The listing builds one solid part. Answer for the finished solid, in the listing's coordinates (mm). Round coordinates to 2 decimals unless told otherwise and drop trailing zeros. Write each loop counter-clockwise with the first axis right and the second up, starting at its lowest first coordinate (ties: lowest second). Pieces come first, ordered by that corner, then holes. Notation, with made-up numbers: (-39, -2) - (13, -2) arc R12 ccw to (13, 3) - close; hole circle Ø7 at (55.25, 30.25). An arc over 180 degrees is marked (long way). Use a Markdown table: item, result. Add a question column.
1) A cutting plane is placed at D-D (x = -40.25). Give the vertices of the cut face in (y, z).
2) A cutting plane is placed at C-C (z = 2.1). State how many separate pieces and enclosed holes the cut face has, then the cut area to 3 significant figures.
3) A cutting plane is placed at B-B (y = -8.75). Give the vertices of the cut face in (x, z).
4) Find the intervals of material crossed by probe 1 along Y at (x, z) = (49, 2.1); probe 2 along Y at (x, z) = (40.25, 2); probe 3 along X at (y, z) = (-7, 1.25), in increasing order. Write a range as from..to.
5) A cutting plane is placed at A-A (x = 57.75). Give the vertices of the cut face in (y, z).
6) Each of these flat-tipped pins is pushed along its axis until it touches: P1, Ø2.5, axis at x = 66.5, y = 0, coming from the -Z side; P2, Ø5, axis at x = -33.84, y = 8.75, coming from the -Z side; P3, Ø1.5, axis at x = -50.5, z = 3.5, coming from the +Y side; P4, Ø1, axis at y = 5, z = 1.5, coming from the +X side. Where does it stop, or does it pass through?
7) Determine the mould class of faces 1 (the flat face through (-1, 0, 0)), 2 (the cylindrical face through (65.634, -8.284, 2.535)), 3 (the flat face through (1, 21, 2)) for opening direction Y: +Y half, -Y half, draft (parallel to the pull), parting line (faces both ways), or undercut.
```python
from build123d import *

# Parameters (mm, degrees)
EXTRUDE_1_DEPTH     = 5
SKETCH_2_R          = 13.5
SKETCH_2_R_2        = 1.55
CUT_EXTRUDE_1_DEPTH = 5


with BuildPart() as part:
    # 草图1 → 凸台-拉伸1 (new body)
    with BuildSketch(Plane.XY):
        with BuildLine():
            Line((-49, -21), (49, -21))
            ThreePointArc((49, -21), (70, 0), (49, 21))
            Line((49, 21), (-49, 21))
            ThreePointArc((-49, 21), (-70, 0), (-49, -21))
        make_face()
    extrude(amount=EXTRUDE_1_DEPTH)

    # 草图2 → 切除-拉伸1 (cut)
    with BuildSketch(Plane.XY.offset(5)):
        with Locations((49, 0)):
            Circle(SKETCH_2_R)
        with Locations((49, 17.5)):
            Circle(SKETCH_2_R_2)
        with Locations((57.75, 15.155444566)):
            Circle(SKETCH_2_R_2)
        with Locations((64.155444566, 8.75)):
            Circle(SKETCH_2_R_2)
        with Locations((66.5, 0)):
            Circle(SKETCH_2_R_2)
        with Locations((64.155444566, -8.75)):
            Circle(SKETCH_2_R_2)
        with Locations((57.75, -15.155444566)):
            Circle(SKETCH_2_R_2)
        with Locations((49, -17.5)):
            Circle(SKETCH_2_R_2)
        with Locations((40.25, -15.155444566)):
            Circle(SKETCH_2_R_2)
        with Locations((33.844555434, -8.75)):
            Circle(SKETCH_2_R_2)
        with Locations((31.5, 0)):
            Circle(SKETCH_2_R_2)
        with Locations((33.844555434, 8.75)):
            Circle(SKETCH_2_R_2)
        with Locations((40.25, 15.155444566)):
            Circle(SKETCH_2_R_2)
    cut_extrude_1 = extrude(amount=-CUT_EXTRUDE_1_DEPTH, mode=Mode.SUBTRACT)

    # 镜向1: 切除-拉伸1 across plane
    add(cut_extrude_1.mirror(Plane(origin=(0, 0, 0), x_dir=(0, 0, 1), z_dir=(1, 0, 0))), mode=Mode.SUBTRACT)


solid = part.part
```
Entries:
| question | item | result |
|---|---|---|
| 1 | outline | (-21, 0) - (-16.71, 0) - (-16.71, 5) - (-21, 5) - close; (-13.61, 0) - (-10.28, 0) - (-10.28, 5) - (-13.61, 5) - close; (10.28, 0) - (13.61, 0) - (13.61, 5) - (10.28, 5) - close; (16.71, 0) - (21, 0) - (21, 5) - (16.71, 5) - close |
| 2 | separate pieces | 1 |
| 2 | enclosed holes | 26 |
| 2 | area | 4,180 mm² |
| 3 | outline | (-68.09, 0) - (-65.71, 0) - (-65.71, 5) - (-68.09, 5) - close; (-62.61, 0) - (-59.28, 0) - (-59.28, 5) - (-62.61, 5) - close; (-38.72, 0) - (-35.39, 0) - (-35.39, 5) - (-38.72, 5) - close; (-32.29, 0) - (32.29, 0) - (32.29, 5) - (-32.29, 5) - close; (35.39, 0) - (38.72, 0) - (38.72, 5) - (35.39, 5) - close; (59.28, 0) - (62.61, 0) - (62.61, 5) - (59.28, 5) - close; (65.71, 0) - (68.09, 0) - (68.09, 5) - (65.71, 5) - close |
| 4 | probe 1 | y = -21..-19.05, -15.95..-13.5, 13.5..15.95, 19.05..21 |
| 4 | probe 2 | y = -21..-16.71, -13.61..-10.28, 10.28..13.61, 16.71..21 |
| 4 | probe 3 | x = -68.8..-60.54, -37.46..37.46, 60.54..68.8 |
| 5 | outline | (-19.09, 0) - (-16.71, 0) - (-16.71, 5) - (-19.09, 5) - close; (-13.61, 0) - (-10.28, 0) - (-10.28, 5) - (-13.61, 5) - close; (10.28, 0) - (13.61, 0) - (13.61, 5) - (10.28, 5) - close; (16.71, 0) - (19.09, 0) - (19.09, 5) - (16.71, 5) - close |
| 6 | P1 | passes through |
| 6 | P2 | stops at z = 0 |
| 6 | P3 | stops at y = 20.99 |
| 6 | P4 | stops at x = 69.51 |
| 7 | face 1 | draft |
| 7 | face 2 | undercut |
| 7 | face 3 | +Y half |
